The listing builds one solid part. Answer for the finished solid, in the listing's coordinates (mm). A direction names the side the tool comes from. Give positions to 0.01 mm unless a question says otherwise; leave off trailing zeros. Loops run counter-clockwise (first coordinate to the right, second up) from the corner with the lowest first, then second, coordinate; pieces in that order, holes last. Notation, with made-up numbers: (46.25, 10) - (100.25, 10) arc R34 ccw to (100.25, 45) - close; hole circle Ø8 at (-19.5, 30). An arc over 180 degrees is marked (long way). Answer as CSV lines item,"result". Start each with the question number.
1) A cutting plane is placed at B-B (z = 9.25). Determine the outline of the cut face in (x, y), and give its area (3 significant figures).
2) Find the intervals of material crossed by line 1 along X through (y, z) = (20.5, 10); line 2 along Z through (x, y) = (65, 83); line 3 along Y through (x, z) = (107, 16.25), in increasing order.
3) For faces 1 (the face through (69, 0, 15)), 2 (the face through (85, 80, 6)), 3 (the face through (62.044, 45, 5)), determine the directions among +Z, -Z, +X, -X, +Y, -Y from which every point of the face is accessible in a straight line to the end or side of a thin tool.
4) Flat-ended cylindrical pins translate along their axes: pin 1 (4 mm diameter, centred on x = 77, y = 48.5, fed in from +Z); pin 2 (2.5 mm diameter, centred on x = 66, z = 16.5, fed in from +Y); pin 3 (6 mm diameter, centred on x = 81, z = 7.5, fed in from -Y). Find the tip coordinate at first contact, or state that the pin passes through.
5) A cutting plane is placed at D-D (x = 89). Determine the outline of the cut face in (y, z).
6) A cutting plane is placed at A-A (y = 48). Determine the outline of the cut face in (x, z), and give its area (3 significant figures).
7) For a pull along X with two mould halves and no side action, classify faces 4 (the face through (94, 36, 7)), 5 (the face through (76, 38, 7)), 6 (the face through (112.044, 45, 5)), 7 (the face through (103, 0, 15)) as pulls with the +X half, pulls with the -X half, needs draft (parallel to the pull), parting line crosses it, or undercut.
8) A cutting plane is placed at C-C (x = 70.5). Determine the outline of the cut face in (y, z), and give its area (3 significant figures).
Autodesk Fusion 360 part; units mm, degrees
sketch "Sketch2" plane through (0, 0, 0) normal (0, 0, 1) x (1, 0, 0) in component "jig"
  line L0 (0, 0) -> (0, 160)
  line L1 (0, 160) -> (134, 160)
  line L2 (134, 160) -> (134, 0)
  line L3 (134, 0) -> (0, 0)
  line L4 (40, 160) -> (58, 160)
  line L5 (58, 160) -> (58, 60)
  line L6 (58, 60) -> (40, 60)
  line L7 (40, 60) -> (40, 160)
  line L8 (76, 0) -> (94, 0)
  line L9 (94, 0) -> (94, 80)
  line L10 (94, 80) -> (76, 80)
  line L11 (76, 80) -> (76, 0)
  line L12 (76, 80) -> (58, 80) construction
  line L13 (0, 160) -> (40, 160)
  line L14 (40, 160) -> (40, 166)
  line L15 (40, 166) -> (0, 166)
  line L16 (0, 166) -> (0, 160)
  line L17 (134, 160) -> (58, 160)
  line L18 (58, 160) -> (58, 166)
  line L19 (58, 166) -> (134, 166)
  line L20 (134, 166) -> (134, 160)
  line L21 (0, 0) -> (76, 0)
  line L22 (76, 0) -> (76, -6)
  line L23 (76, -6) -> (0, -6)
  line L24 (0, -6) -> (0, 0)
  line L25 (134, 0) -> (94, 0)
  line L26 (94, 0) -> (94, -6)
  line L27 (94, -6) -> (134, -6)
  line L28 (134, -6) -> (134, 0)
  dimension "d18" = 18
  dimension "d21" = 80
  dimension "d22" = 60
  dimension "d23" = 80
  dimension "d25" = 40
  dimension "d27" = 40
  dimension "d28" = 6
  dimension "d29" = 6
extrude "Extrude1" add sketch "Sketch2" along normal blind 12 contours L0 L1 L2 L3 L5 L6 L7 L9 L10 L11 L13 L17 L21 L25 in component "jig"
extrude "Extrude2" add sketch "Sketch2" along normal blind 18 contours L3 L21 L22 L23 L24 | L1 L13 L14 L15 L16 | L3 L25 L26 L27 L28 | L1 L17 L18 L19 L20 in component "jig"
sketch "Sketch3" plane through (0, 0, 0) normal (-1, 0, 0) x (0, -1, 0) in component "jig"
  line L0 (-166, 0) -> (6, 0)
  line L1 (6, 0) -> (6, 18)
  line L2 (6, 18) -> (0, 18)
  line L3 (0, 18) -> (0, 12)
  line L4 (0, 12) -> (-160, 12)
  line L5 (-160, 12) -> (-160, 18)
  line L6 (-160, 18) -> (-166, 18)
  line L7 (-166, 18) -> (-166, 0)
  line L8 (-160, 13) -> (-160.4879, 12.5121)
  line L9 (-160.2757, 12) -> (-160, 12)
  line L10 (-160, 13) -> (-160, 12)
  arc A0 (-160.4879, 12.5121) -> (-160.2757, 12) centre (-160.2757, 12.3) ccw
  line L11 (0, 12) -> (0.2757, 12)
  line L12 (0.4879, 12.5121) -> (0, 13)
  line L13 (0, 12) -> (0, 13)
  arc A1 (0.2757, 12) -> (0.4879, 12.5121) centre (0.2757, 12.3) ccw
  dimension "d34" = 1
  dimension "d35" = 0.3
  dimension "d36" = 45
  dimension "d37" = 1
  dimension "d38" = 45
  dimension "d39" = 0.3
extrude "Extrude3" cut sketch "Sketch3" against normal up to surface (134 mm away) contours L5 L8 L9 L10 A0 | L3 L11 L12 L13 A1 in component "jig"
box "BoxPrimitive1" cut length 30 width 50 height -100 placed x (0, 0, -1) y (1, 0, 0) z (0, -1, 0) at (62.0445, -6, 30) keep common part in component "jig"
component "jig" placed x (1, 0, 0) y (0, 1, 0) z (0, 0, 1) at (0, 0, 0)
equation "stockW = 200 mm"
equation "stockH = 120 mm"
equation "stockT = 18 mm"
equation "lipT = stockT / 3"
equation "lipH = lipT"
equation "jigT = 12 mm"
equation "stock2H = 160 mm"
equation "d18 = stockT"
equation "d21 = stock2H / 2"
equation "d22 = stockH / 2"
equation "d23 = stock2H / 2"
equation "baseMargin = 40 mm"
equation "d25 = baseMargin"
equation "d27 = baseMargin"
equation "d28 = lipT"
equation "d29 = lipT"
equation "d30 = jigT"
equation "d32 = jigT + lipT"
Ans:
1,outline,"(62.04, -6) - (76, -6) - (76, 80) - (94, 80) - (94, -6) - (112.04, -6) - (112.04, 94) - (62.04, 94) - close"
1,area,"3,450 mm2"
2,line 1,"62.04 to 76, 94 to 112.04"
2,line 2,"0 to 12"
2,line 3,"-6 to 0"
3,face 1,"+Z, +X, -X, +Y"
3,face 2,"+Z, -Z, -Y"
3,face 3,"+Z, -Z, -X, +Y, -Y"
4,pin 1,"z = 12"
4,pin 2,"y = 0"
4,pin 3,"y = 80"
5,outline,"(80, 0) - (94, 0) - (94, 12) - (80, 12) - close"
6,outline,"(62.04, 0) - (76, 0) - (76, 12) - (62.04, 12) - close; (94, 0) - (112.04, 0) - (112.04, 12) - (94, 12) - close"
6,area,"384 mm2"
7,face 4,"undercut"
7,face 5,"undercut"
7,face 6,"pulls with the +X half"
7,face 7,"needs draft"
8,outline,"(-6, 0) - (94, 0) - (94, 12) - (-0.28, 12) arc R0.3 cw to (-0.49, 12.51) - (0, 13) - (0, 18) - (-6, 18) - close"
8,area,"1,240 mm2"
